Verification items for the finished model (mm, model axes). Round coordinates to 2 decimals unless told otherwise and drop trailing zeros. Order: outer loops, then holes, each group sorted by start corner. A loop starts at its lowest first (then second) coordinate and runs counter-clockwise, first axis right, second up. Notation, with made-up numbers: (49, 75) -> (80, 75) arc R21 ccw to (80, 105) -> close; hole circle Ø2 at (8.5, 70). An arc over 180 degrees is marked (long way). Write item = value, one per line. Start each with the question number.
from build123d import *

# Parameters (mm, degrees)
F0_R     = 10
F1_DEPTH = 500


with BuildPart() as f1:
    # F0 (on Right) → F1 (new body)
    with BuildSketch(Plane.YZ):
        Circle(F0_R)
    extrude(amount=F1_DEPTH)

    # F2 (on Front) → F3 (revolve)
    with BuildSketch(Plane.XZ):
        Polygon((-4.5, -5), (0, -9.90314), (0, 0), (-4.5, 0), align=None)
    revolve(axis=Axis((-2.25, 0, 0), (1, 0, 0)))

    # F4 (on Front) → F5 (revolve, cut)
    with BuildSketch(Plane.XZ):
        with BuildLine():
            Line((-5, 0), (0, 0))
            ThreePointArc((0, 0), (-1.464466, 3.535534), (-5, 5))
            Line((-5, 5), (-5, 0))
        make_face()
    revolve(axis=Axis((-7.712245, 0, 0), (-1, 0, 0)), mode=Mode.SUBTRACT)

    # F6 (on Front) → F7 (revolve)
    with BuildSketch(Plane.XZ):
        with BuildLine():
            Line((500, 0), (510, 0))
            ThreePointArc((510, 0), (507.071068, 7.071068), (500, 10))
            Line((500, 10), (500, 0))
        make_face()
    revolve(axis=Axis((505, 0, 0), (1, 0, 0)))


solid = f1.part
(1) Cross-section at A-A (x = 63.5). Enter the section's corners in (y, z).
(2) Depth check by flat-ended pin: pin 1 (3 mm diameter, centred on y = -2.5, z = 2.5, fed in from -X); pin 2 (6 mm diameter, centred on y = 1, z = 6, fed in from +X); pin 3 (1.5 mm diameter, centred on x = 307.5, z = 1, fed in from -Y); pin 4 (1.5 mm diameter, centred on x = 95.5, y = 4.5, fed in from -Z). Enter the tip coordinate at first touch or a pass-through.
(3) Scan lines: line 1 along Y through (x, z) = (157, -1.5); line 2 along Z through (x, y) = (460.5, 0.25); line 3 along Y through (x, z) = (164, 0.75). Record each from-to range of solid material in increasing order. Write a range as from..to.
Outcome:
q1.outline = circle Ø20 at (0, 0)
q2.pin_1 = -4.5
q2.pin_2 = 509.51
q2.pin_3 = -10
q2.pin_4 = -9.27
q3.line_1 = -9.89..9.89
q3.line_2 = -10..10
q3.line_3 = -9.97..9.97
